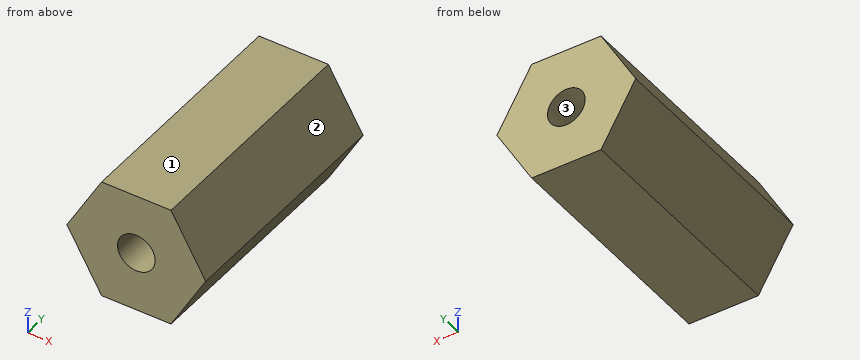
from build123d import *

# Parameters (mm, degrees)
BOSS_EXTRUDE1_DEPTH     = 12.5
CUT_EXTRUDE1_DEPTH      = 16.812644729
CUT_EXTRUDE1_DEPTH_BACK = 16.812644729
SKETCH3_R               = 1.985


with BuildPart() as part:
    # Sketch2 → Boss-Extrude1 (new, symmetric)
    with BuildSketch(Plane(origin=(0, 0, 0), x_dir=(1, 0, 0), z_dir=(0, 1, 0))):
        Polygon((7.320801413, 0), (3.660400707, 6.34), (-3.660400707, 6.34), (-7.320801413, 0), (-3.660400707, -6.34), (3.660400707, -6.34), align=None)
    extrude(amount=BOSS_EXTRUDE1_DEPTH, both=True)

    # Sketch3 → Cut-Extrude1 (cut, two sides: drawn at the far end of the back side and taken through both)
    with BuildSketch(Plane(origin=(0, 0, 0), x_dir=(1, 0, 0), z_dir=(0, 1, 0)).offset(-CUT_EXTRUDE1_DEPTH_BACK)):
        with Locations(Location((0, 0, 0), (0, 0, 270))):
            Circle(SKETCH3_R)
    extrude(amount=CUT_EXTRUDE1_DEPTH + CUT_EXTRUDE1_DEPTH_BACK, mode=Mode.SUBTRACT)


solid = part.part
Geometry check sheet. Reference: the model listing, model coordinates, mm. Face numbers are marked on the shaded views. Round coordinates to 2 decimals unless told otherwise and drop trailing zeros. Order: outer loops, then holes, each group sorted by start corner. A loop starts at its lowest first (then second) coordinate and runs counter-clockwise, first axis right, second up. Notation, with made-up numbers: M -32,23.5 L -4,23.5 A9 cw -4,33.5 Z; hole C -36,40 d1. An arc over 180 degrees is marked long. Write each question's results on one line, items separated by ' | '. Start each with the question number.
1. Draft check along X on the marked faces 1, 2 and 3. Enter one of: pulls with the +X half, pulls with the -X half, needs draft (parallel to the pull), parting line crosses it, or undercut.
2. Cross-section at B-B on x = 0. Record the boundary of the cut face in (y, z) (3 decimals), plus the area to 3 significant figures.
3. Material ranges on L1, parallel to Z at x = 0, y = 9 (3 decimals); L2, parallel to X at y = -9.5, z = 0.25; L3, parallel to X at y = 6, z = 1.25, recorded low to high. Write a range as from..to.
4. Go/stop test with flat-tipped pins: P1, Ø1.5, axis at y = 8.5, z = -5, coming from the +X side; P2, Ø1.5, axis at y = -1.5, z = 4.5, coming from the -X side; P3, Ø4, axis at y = 8, z = -3.5, coming from the -X side. Record where each tip stops, or that it passes through.
5. Cross-section at A-A on y = 6.5. Record the boundary of the cut face in (x, z) (3 decimals), plus the area to 3 significant figures.
6. Cross-section at D-D on x = -4.5. Record the boundary of the cut face in (y, z).
7. Cross-section at C-C on z = 3.5. Record the boundary of the cut face in (x, y).
Resolved:
1) face 1: needs draft | face 2: pulls with the +X half | face 3: undercut
2) outline: M -12.5,-6.34 L 12.5,-6.34 L 12.5,-1.985 L -12.5,-1.985 Z; M -12.5,1.985 L 12.5,1.985 L 12.5,6.34 L -12.5,6.34 Z | area: 218 mm2
3) L1: -6.34..-1.985, 1.985..6.34 | L2: -7.18..-1.97, 1.97..7.18 | L3: -6.6..-1.54, 1.54..6.6
4) P1: x = 4.87 | P2: x = -5.16 | P3: x = -6.45
5) outline: M -7.321,0 L -3.66,-6.34 L 3.66,-6.34 L 7.321,0 L 3.66,6.34 L -3.66,6.34 Z; hole C 0,0 d3.97 | area: 127 mm2
6) outline: M -12.5,-4.89 L 12.5,-4.89 L 12.5,4.89 L -12.5,4.89 Z
7) outline: M -5.3,-12.5 L 5.3,-12.5 L 5.3,12.5 L -5.3,12.5 Z
